Geometry check sheet. Reference: the model listing, model coordinates, mm. A direction names the side the tool comes from. Coordinates: 2 decimals unless noted, no trailing zeros. Write each loop counter-clockwise with the first axis right and the second up, starting at its lowest first coordinate (ties: lowest second). Pieces come first, ordered by that corner, then holes. Notation, with made-up numbers: M -18.75,-25 L 15.25,-25 A14 ccw 15.25,-10 Z; hole C 69,60.25 d10. An arc over 180 degrees is marked long. Answer as a JSON object with one key per item and string values. Group by question number.
Autodesk Inventor part; units mm, degrees
ref_plane "YZ Plane" through (0, 0, 0) normal (1, 0, 0) x (0, 1, 0)
ref_plane "XZ Plane" through (0, 0, 0) normal (0, 1, 0) x (-1, 0, 0)
ref_plane "XY Plane" through (0, 0, 0) normal (0, 0, 1) x (1, 0, 0)
sketch "スケッチ1" plane through (0, 0, 0) normal (0, 0, 1) x (1, 0, 0)
  circle A0 centre (0, 0) radius 3
  dimension "d0" = 6
extrude "押し出し1" add sketch "スケッチ1" along normal blind 40
hole "穴1" at (0, 0, 0) direction (0, 0, 1) diameter 3 depth 6 tip angle 118
sketch "スケッチ2" plane through (0, 0, 40) normal (0, 0, 1) x (1, 0, 0)
  circle A0 centre (0, 0) radius 3
hole "穴2" at (0, 0, 40) direction (0, 0, -1) diameter 3 depth 6 tip angle 118
properties part number "スペーサ　m3-l40" material "アルミニウム 2014-T4"
1) Section check B-B (x = -2.4). Record the cut outline in (y, z).
2) Set-up check for faces 5 (the cylindrical face through (-0.07, 1.5, 36.96)), 6 (the flat face through (1.3, -1.3, 0)), 7 (the cylindrical face through (-0.07, -1.5, 3.04)): record each of +Z, -Z, +X, -X, +Y, -Y from which the full face is reachable in a straight line by a thin tool's end or side.
3) Draft check along Y on faces 1 (the conical face through (-0.254, -0.056, 6.745)), 2 (the conical face through (-0.231, -0.12, 33.255)), 3 (the cylindrical face through (-3, 0, 20)), 4 (the flat face through (1.3, -1.3, 40)). Enter one of: +Y half, -Y half, draft (parallel to the pull), parting line (faces both ways), or undercut.
4) Material ranges on probe 1 along Y at (x, z) = (0, 38.1); probe 2 along Y at (x, z) = (2.6, 19); probe 3 along X at (y, z) = (-0.1, 27.5), recorded low to high. Write a range as [from, to].
5) Section check A-A (z = 18.5). Record the cut outline in (x, y), then the cut area to 3 significant figures.
6) Go/stop test with flat-tipped pins: pin 1 Ø2 at (x, y) = (1.5, -0.5) entering from -Z; pin 2 Ø1.5 at (y, z) = (-2, 33.5) entering from +X. Record where each tip stops, or that it passes through.
Entries:
{
 "1": {"outline": "M -1.8,0 L 1.8,0 L 1.8,40 L -1.8,40 Z"},
 "2": {"face 5": "+Z", "face 6": "-Z, +X, -X, +Y, -Y", "face 7": "-Z"},
 "3": {"face 1": "undercut", "face 2": "undercut", "face 3": "parting line", "face 4": "draft"},
 "4": {"probe 1": "[-3, -1.5], [1.5, 3]", "probe 2": "[-1.5, 1.5]", "probe 3": "[-3, 3]"},
 "5": {"outline": "C 0,0 d6", "area": "28.3 mm^2"},
 "6": {"pin 1": "z = 0", "pin 2": "x = 2.73"}
}
